The figure shows three views and two pictorial views of one solid part (mm, origin at its lowest corner). Answer the questions. Give positions to 0.01 mm unless a question says otherwise; leave off trailing zeros. Order: outer loops, then holes, each group sorted by start corner. A loop starts at its lowest first (then second) coordinate and runs counter-clockwise, first axis right, second up. Notation, with made-up numbers: (-4, 61.5) - (8, 61.5) arc R21 ccw to (8, 82.5) - close; hole circle Ø3 at (54.25, -12.75). An arc over 180 degrees is marked (long way). Answer as CSV lines item,"result". Start each with the question number.
1. Flat-ended cylindrical pins translate along their axes: pin 1 (0.9 mm diameter, centred on y = 1.5, z = 28, fed in from +X); pin 2 (1.5 mm diameter, centred on y = 1, z = 67, fed in from +X); pin 3 (1 mm diameter, centred on x = 24.5, z = 73, fed in from +Y); pin 4 (1.5 mm diameter, centred on y = 2, z = 38.5, fed in from +X). Find the tip coordinate at first contact, or state that the pin passes through.
2. Section C-C on y = 0.5 is taken. Give the vertices of the cut face in (x, z), and give its area (3 significant figures).
3. Section D-D on x = 31 is taken. Give the vertices of the cut face in (y, z), and give its area (3 significant figures).
4. Section B-B on x = 19.5 is taken. Give the vertices of the cut face in (y, z).
5. Section A-A on z = 38 is taken. Give the vertices of the cut face in (x, y), and give its area (3 significant figures).
6. Consider line 1 along Z through (x, y) = (18.5, 1.6); line 2 along X through (y, z) = (0.55, 89.5); line 3 along Z through (x, y) = (32.5, 1.9). Determine where each line is inside the solid, lowest interval first. Write a range as [from, to].
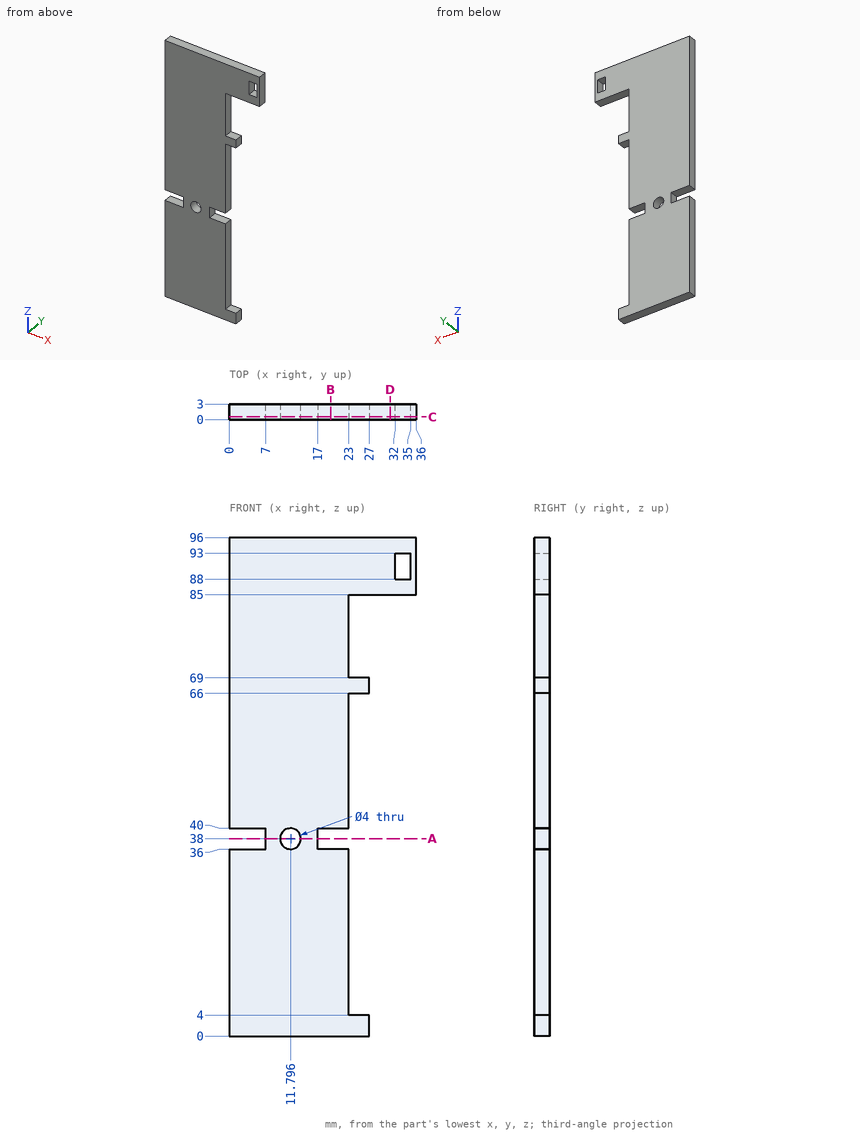
Checks:
1,pin 1,"stops at x = 23"
1,pin 2,"stops at x = 27"
1,pin 3,"passes through"
1,pin 4,"stops at x = 17"
2,outline,"(0, 0) - (27, 0) - (27, 4) - (23, 4) - (23, 36) - (17, 36) - (17, 40) - (23, 40) - (23, 66) - (27, 66) - (27, 69) - (23, 69) - (23, 85) - (36, 85) - (36, 96) - (0, 96) - (0, 40) - (7, 40) - (7, 36) - (0, 36) - close; hole circle Ø4 at (11.8, 38); hole (32, 88) - (35, 88) - (35, 93) - (32, 93) - close"
2,area,"2,300 mm²"
3,outline,"(0, 85) - (3, 85) - (3, 96) - (0, 96) - close"
3,area,"33.0 mm²"
4,outline,"(0, 0) - (3, 0) - (3, 36) - (0, 36) - close; (0, 40) - (3, 40) - (3, 96) - (0, 96) - close"
5,outline,"(7, 0) - (9.8, 0) - (9.8, 3) - (7, 3) - close; (13.8, 0) - (17, 0) - (17, 3) - (13.8, 3) - close"
5,area,"18.0 mm²"
6,line 1,"z = [0, 36], [40, 96]"
6,line 2,"x = [0, 32], [35, 36]"
6,line 3,"z = [85, 88], [93, 96]"
